```python
from build123d import *

# Parameters (mm, degrees)
BOSS_EXTRUDE1_DEPTH = 62
BOSS_EXTRUDE2_DEPTH = 5


with BuildPart() as part:
    # Sketch1 → Boss-Extrude1 (new body)
    with BuildSketch(Plane(origin=(0, 0, 0), x_dir=(1, 0, 0), z_dir=(0, 1, 0))):
        with BuildLine():
            Line((-2.5, -12), (-2.5, 12))
            ThreePointArc((-2.5, 12), (0, 14.5), (2.5, 12))
            Line((2.5, 12), (2.5, -12))
            ThreePointArc((2.5, -12), (0, -14.5), (-2.5, -12))
        make_face()
    extrude(amount=-BOSS_EXTRUDE1_DEPTH)

    # Sketch2 → Boss-Extrude2 (add)
    with BuildSketch(Plane(origin=(0, 0, 0), x_dir=(1, 0, 0), z_dir=(0, 1, 0))):
        with BuildLine():
            Line((4, -12), (4, 12))
            ThreePointArc((4, 12), (0, 16), (-4, 12))
            Line((-4, 12), (-4, -12))
            ThreePointArc((-4, -12), (0, -16), (4, -12))
        make_face()
    extrude(amount=-BOSS_EXTRUDE2_DEPTH)


solid = part.part
```
For this review, take the finished solid that the model builds, in its own axes (mm). A direction names the side the tool comes from. Round coordinates to 2 decimals unless told otherwise and drop trailing zeros. Loops run counter-clockwise (first coordinate to the right, second up) from the corner with the lowest first, then second, coordinate; pieces in that order, holes last.
(1) Wall thickness on line 1 along Y through (x, z) = (3.25, -12); line 2 along X through (y, z) = (-44.5, 2); line 3 along Z through (x, y) = (0.25, -35): over which ranges is each line inside the solid? List them lowest first.
Returned:
line 1: y = -5 to 0
line 2: x = -2.5 to 2.5
line 3: z = -14.49 to 14.49
(2) We need section A-A (x = 0). Give the boundary of the cut face in (y, z), plus the area to 3 significant figures.
Returned:
outline: (-62, -14.5) - (-5, -14.5) - (-5, -16) - (0, -16) - (0, 16) - (-5, 16) - (-5, 14.5) - (-62, 14.5) - close
area: 1,810 mm2
(3) Tool access review of faces 1 (the cylindrical face through (-0.1, -33.1, -14.5)), 2 (the cylindrical face through (0.1, -33.1, 14.5)), 3 (the flat face through (2.5, -33, 0)), 4 (the flat face through (-2.5, -33, 0)): name each direction out of +Z, -Z, +X, -X, +Y, -Y from which nothing blocks a thin tool from reaching the whole face with its end or side.
Returned:
face 1: -Z, -Y
face 2: +Z, -Y
face 3: +Z, -Z, +X, -Y
face 4: +Z, -Z, -X, -Y
(4) We need section C-C (y = -47). Give the boundary of the cut face in (x, z).
Returned:
outline: (-2.5, -12) arc R2.5 ccw to (2.5, -12) - (2.5, 12) arc R2.5 ccw to (-2.5, 12) - close
(5) We need section B-B (z = 1.5). Give the boundary of the cut face in (x, y).
Returned:
outline: (-4, -5) - (-2.5, -5) - (-2.5, -62) - (2.5, -62) - (2.5, -5) - (4, -5) - (4, 0) - (-4, 0) - close
(6) Clearance check with flat-ended pins moving along their axes: P1, Ø7, axis at y = -42.5, z = -1.5, coming from the +X side; P2, Ø4, axis at x = 0.5, y = -43, coming from the -Z side; P3, Ø6, axis at y = -30.5, z = -2.5, coming from the -X side. State where each tip first meets the part, or that it passes through.
Returned:
P1: stops at x = 2.5
P2: stops at z = -14.5
P3: stops at x = -2.5
